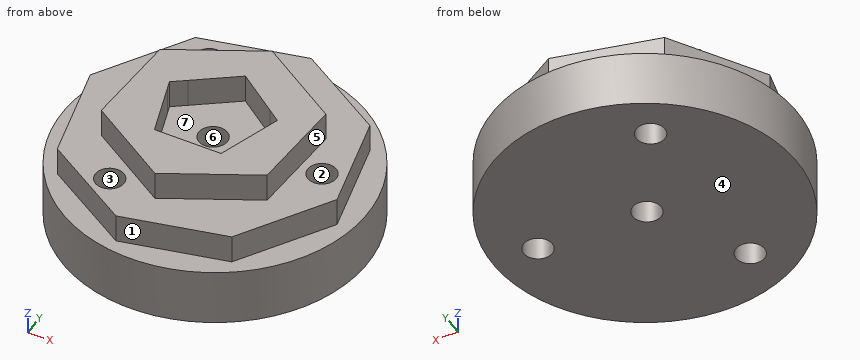
```python
from build123d import *

# Parameters (mm, degrees)
F0_R       = 33.7251473282
F5_DEPTH   = 12.7
F6_DEPTH   = 25.4
F7_DEPTH   = 19.05
F8_D       = 6.35
F8_ON_F4_D = 6.35


with BuildPart() as f5:
    # F0 (on Top) → F5 (new body)
    with BuildSketch(Plane.XY):
        with Locations((-39.3072403967, -35.1206697524)):
            Circle(F0_R)
    extrude(amount=F5_DEPTH)

    # F1 (on face) → F6 (join)
    with BuildSketch(Plane.XY):
        Polygon((-20.2098016627, -24.7553280585), (-38.8420633972, -13.0248842761), (-30.4153332648, -29.0032569477), (-27.5516730192, -31.0838279019), (-28.2250702608, -33.1563315064), (-21.0525331088, -46.7565619417), align=None)
        Polygon((-30.4153332648, -29.0032569477), (-38.8420633972, -13.0248842761), (-48.8573559288, -28.9328546186), (-39.6847948432, -22.2685988992), align=None)
        Polygon((-48.8573559288, -28.9328546186), (-38.8420633972, -13.0248842761), (-58.3170565776, -23.2956743769), (-59.1597880237, -45.2969082601), (-51.2710974395, -32.7667644367), (-51.8179166672, -31.0838279019), align=None)
        Polygon((-21.0525331088, -46.7565619417), (-28.2250702608, -33.1563315064), (-32.1861131663, -45.3471680467), (-47.1834765201, -45.3471680467), (-51.2710974395, -32.7667644367), (-59.1597880237, -45.2969082601), align=None)
        Polygon((-40.5275262892, -57.0273520425), (-21.0525331088, -46.7565619417), (-59.1597880237, -45.2969082601), align=None)
    extrude(amount=F6_DEPTH)

    # F2 (on Top) → F7 (join)
    with BuildSketch(Plane.XY):
        Polygon((-14.6972839647, -16.8937072017), (-34.8278614766, -4.542624592), (-57.7958636127, -10.0435581916), (-70.1469462224, -30.1741357035), (-64.6460126228, -53.1421378396), (-44.5154351109, -65.4932204493), (-21.5474329747, -59.9922868497), (-9.1963503651, -39.8617093378), align=None)
    extrude(amount=F7_DEPTH)

    # F8 (through all)
    with Locations(Plane(origin=(0, 0, 0), x_dir=(1, 0, 0), z_dir=(0, 0, -1))):
        with Locations((-39.8223698139, 34.9703021348)):
            Hole(F8_D / 2)

    # F8 on F4 (through all)
    with Locations(Plane(origin=(0, 0, 0), x_dir=(1, 0, 0), z_dir=(0, 0, -1))):
        with Locations((-52.2050820291, 14.4365634769), (-51.214001947, 56.08092756), (-15.6444647677, 34.4004449901)):
            Hole(F8_ON_F4_D / 2)


solid = f5.part
```
Geometry check sheet. Reference: the model listing, model coordinates, mm. Face numbers are marked on the shaded views. A direction names the side the tool comes from. Give positions to 0.01 mm unless a question says otherwise; leave off trailing zeros. Loops run counter-clockwise (first coordinate to the right, second up) from the corner with the lowest first, then second, coordinate; pieces in that order, holes last. Notation, with made-up numbers: M 30,6.5 L 38,6.5 A9 ccw 38,17.5 Z; hole C -12.75,-31.5 d2. An arc over 180 degrees is marked long. Write item = value, one per line.
(1) Gauge pin test, flat ends, axial feed: pin 1 Ø8 at (x, z) = (-14.5, 9.5) entering from +Y; pin 2 Ø1.5 at (y, z) = (-58, 6.5) entering from +X; pin 3 Ø1 at (x, y) = (-43, -41) entering from -Z; pin 4 Ø4 at (x, y) = (-51.21, -56.08) entering from +Z. Record the tip position at first contact, or that the pin passes through.
Answer below:
pin_1 = -8.58
pin_2 = -13.86
pin_3 = 0
pin_4 = through
(2) Sectioned sample at B-B, the plane y = -5.5. Record the cut outline in (x, z).
Answer below:
outline = M -55.43,0 L -23.18,0 L -23.18,12.7 L -33.27,12.7 L -33.27,19.05 L -38.83,19.05 L -38.83,12.7 L -55.43,12.7 Z
(3) Sectioned sample at C-C, the plane x = -67.5. Record the cut outline in (y, z).
Answer below:
outline = M -53.63,0 L -16.61,0 L -16.61,12.7 L -25.86,12.7 L -25.86,19.05 L -41.23,19.05 L -41.23,12.7 L -53.63,12.7 Z
(4) Material ranges on line 1 (Z direction, x = -43, y = -44.5); line 2 (X direction, y = -33, z = 9); line 3 (Y direction, x = -17, z = 10), recorded low to high. Write a range as [from, to].
Answer below:
line_1 = [0, 19.05]
line_2 = [-72.97, -42.31], [-37.33, -18.49], [-12.8, -5.65]
line_3 = [-60.41, -37.27], [-31.53, -9.83]
(5) Release check for a two-part mould opening along X. For the marked faces 1, 2, 3 and 4 record: released by +X, released by -X, zero draft, split by the parting line, or undercut.
Answer below:
face_1 = released by +X
face_2 = undercut
face_3 = undercut
face_4 = zero draft
(6) Sectioned sample at A-A, the plane z = 14.75. Record the cut outline in (x, y) (3 decimals), plus the area to 3 significant figures.
Answer below:
outline = M -70.147,-30.174 L -64.646,-53.142 L -44.515,-65.493 L -21.547,-59.992 L -9.196,-39.862 L -14.697,-16.894 L -34.828,-4.543 L -57.796,-10.044 Z; hole C -52.205,-14.437 d6.35; hole C -51.214,-56.081 d6.35; hole C -39.822,-34.97 d6.35; hole C -15.644,-34.4 d6.35
area = 2,570 mm2
(7) Sectioned sample at D-D, the plane y = -39. Record the cut outline in (x, z), plus the area to 3 significant figures.
Answer below:
outline = M -72.81,0 L -5.81,0 L -5.81,12.7 L -9.4,12.7 L -9.4,19.05 L -20.76,19.05 L -20.76,25.4 L -30.12,25.4 L -30.12,19.05 L -49.25,19.05 L -49.25,25.4 L -58.92,25.4 L -58.92,19.05 L -68.03,19.05 L -68.03,12.7 L -72.81,12.7 Z
area = 1,340 mm2
(8) Tool access check on the marked faces 5, 6 and 7. Record the directions out of +Z, -Z, +X, -X, +Y, -Y that give a thin tool (end or side, any length) a straight path to the whole face; none if there is none.
Answer below:
face_5 = +Z, +X, -Y
face_6 = +Z, -Z
face_7 = +Z
